Geometry: see drawing. Coordinates: mm, zero at the bounding-box minimum. A direction names the side the tool comes from. Give positions to 0.01 mm unless a question says otherwise; leave off trailing zeros. Loops run counter-clockwise (first coordinate to the right, second up) from the corner with the lowest first, then second, coordinate; pieces in that order, holes last. Notation, with made-up numbers: (34, 69.25) -> (65, 69.25) arc R31 cw to (65, 93.25) -> close; hole circle Ø10 at (71.25, 37). An arc over 180 degrees is marked (long way). Answer in a Markdown table with one row per item. Add a question column.
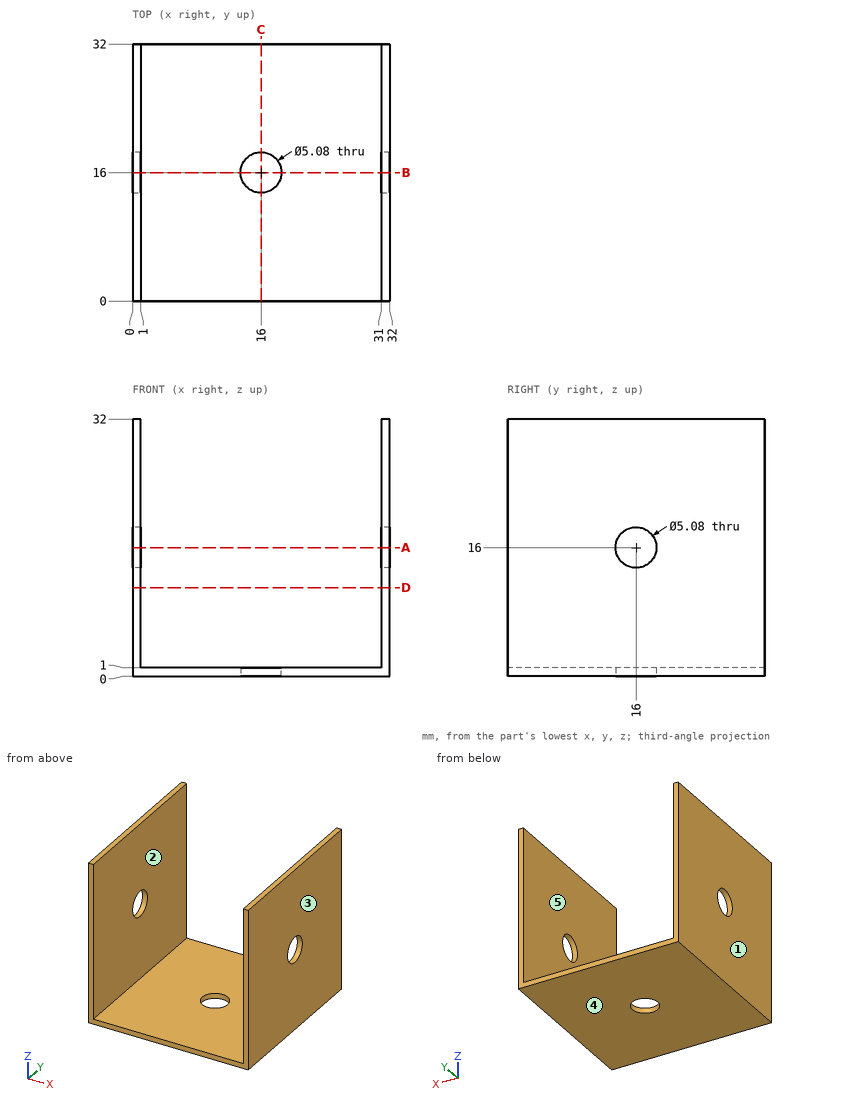
1) Pin query (flat end, axial travel): pin 1 (3 mm diameter, centred on x = 16, y = 16, fed in from +Z); pin 2 (4 mm diameter, centred on x = 17, y = 10.5, fed in from +Z). Return the tip coordinate at first contact, or that it passes through.
2) Section A-A on z = 16. Output: boundary loops of the cut face in (x, y).
3) Reachability of the marked faces 1 and 2 from +Z, -Z, +X, -X, +Y, -Y: full face, straight path, thin tool, end or side. Return the list, or none.
4) Section C-C on x = 16. Output: boundary loops of the cut face in (y, z).
5) Pull-direction query (X, two-part tool) for the marked faces 3, 4 and 5; classes: +X half, -X half, draft (parallel to the pull), parting line (faces both ways), or undercut.
6) Section D-D on z = 11. Output: boundary loops of the cut face in (x, y).
7) Section B-B on y = 16. Output: boundary loops of the cut face in (x, z), and give its area (3 significant figures).
8) Material intervals for line 1 along Z through (x, y) = (31.45, 16); line 2 along X through (y, z) = (26, 15); line 3 along Z through (x, y) = (23.5, 8), sorted ascending.
Working result:
| question | item | result |
|---|---|---|
| 1 | pin 1 | passes through |
| 1 | pin 2 | stops at z = 1 |
| 2 | outline | (0, 0) -> (1, 0) -> (1, 13.46) -> (0, 13.46) -> close; (0, 18.54) -> (1, 18.54) -> (1, 32) -> (0, 32) -> close; (31, 0) -> (32, 0) -> (32, 13.46) -> (31, 13.46) -> close; (31, 18.54) -> (32, 18.54) -> (32, 32) -> (31, 32) -> close |
| 3 | face 1 | +Z, -Z, -X, +Y, -Y |
| 3 | face 2 | +Z, +Y, -Y |
| 4 | outline | (0, 0) -> (13.46, 0) -> (13.46, 1) -> (0, 1) -> close; (18.54, 0) -> (32, 0) -> (32, 1) -> (18.54, 1) -> close |
| 5 | face 3 | +X half |
| 5 | face 4 | draft |
| 5 | face 5 | undercut |
| 6 | outline | (0, 0) -> (1, 0) -> (1, 32) -> (0, 32) -> close; (31, 0) -> (32, 0) -> (32, 32) -> (31, 32) -> close |
| 7 | outline | (0, 0) -> (13.46, 0) -> (13.46, 1) -> (1, 1) -> (1, 13.46) -> (0, 13.46) -> close; (0, 18.54) -> (1, 18.54) -> (1, 32) -> (0, 32) -> close; (18.54, 0) -> (32, 0) -> (32, 13.46) -> (31, 13.46) -> (31, 1) -> (18.54, 1) -> close; (31, 18.54) -> (32, 18.54) -> (32, 32) -> (31, 32) -> close |
| 7 | area | 78.8 mm2 |
| 8 | line 1 | z = 0 to 13.46, 18.54 to 32 |
| 8 | line 2 | x = 0 to 1, 31 to 32 |
| 8 | line 3 | z = 0 to 1 |
